Read the model definition and answer for the solid it produces. Units are mm, in the model's axes. Face numbers are marked on the shaded views. A direction names the side the tool comes from. Coordinates: 2 decimals unless noted, no trailing zeros. Order: outer loops, then holes, each group sorted by start corner. A loop starts at its lowest first (then second) coordinate and runs counter-clockwise, first axis right, second up. Notation, with made-up numbers: (-28.5, 89) -> (18.5, 89) arc R14 cw to (18.5, 104) -> close; hole circle Ø5 at (14.5, -37.75). An arc over 180 degrees is marked (long way). Answer as a JSON object with one key per item and string values. Group by question number.
1) Consider L1, parallel to Y at x = 0, z = 6; L2, parallel to X at y = 0, z = 3; L3, parallel to Z at x = -0.75, y = -2. Determine where each line is inside the solid, lowest interval first.
2) Section D-D on z = 11 is taken. Determine the outline of the cut face in (x, y), and give its area (3 significant figures).
3) A tool of negligible diameter and unlimited length cuts with its end or side. For the marked faces 4, 5 and 6, from which of +Z, -Z, +X, -X, +Y, -Y can it reach the whole face along a straight path? Write none if from no direction.
4) Given pin 1 (6 mm diameter, centred on x = 3, z = 6.5, fed in from +Y); pin 2 (7 mm diameter, centred on y = -1.5, z = 20.5, fed in from -X); pin 3 (1.5 mm diameter, centred on y = -8.5, z = 13.5, fed in from -X); pin 4 (1.5 mm diameter, centred on x = -4, y = -9.5, fed in from +Z), each flat-ended and moving along its own axis, determine where each tip first touches the part or whether it passes through.
5) Section C-C on x = 0 is taken. Determine the outline of the cut face in (y, z).
6) Section B-B on z = 19.5 is taken. Determine the outline of the cut face in (x, y).
7) Determine the mould class of the marked faces 1, 2 and 3 for opening direction X: released by +X, released by -X, zero draft, split by the parting line, or undercut.
8) Section A-A on y = 0 is taken. Determine the outline of the cut face in (x, z), and give its area (3 significant figures).
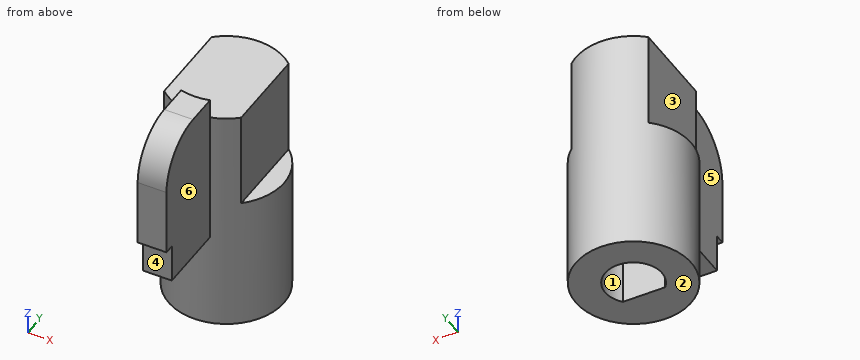
from build123d import *

# Parameters (mm, degrees)
F0_R      = 6
F1_DEPTH  = 10
F2_R      = 6
F3_DEPTH  = 6
F5_DEPTH  = 16
F7_DEPTH  = 8
F8_W      = 1
F8_H      = 4
F9_DEPTH  = 7.501
F10_DEPTH = 2


# Not quite as in the source:
# - a feature names something its author has since deleted; it is built from what else it names


with BuildPart() as f1:
    # F0 (on Top) → F1 (new body)
    with BuildSketch(Plane.XY):
        Circle(F0_R)
        with BuildLine():
            ThreePointArc((-2.1988001779, -1.9666666667), (0, 2.95), (2.1988001779, -1.9666666667))
            Line((2.1988001779, -1.9666666667), (-2.1988001779, -1.9666666667))
        make_face(mode=Mode.SUBTRACT)
    extrude(amount=F1_DEPTH)

    # F2 (on face) → F3 (join)
    with BuildSketch(Plane.XY.offset(10)):
        Circle(F2_R)
    extrude(amount=F3_DEPTH)



with BuildPart() as f5:
    # F4 (on face) → F5 (new body)
    with BuildSketch(Plane.XY.offset(10)):
        with BuildLine():
            ThreePointArc((1.5, -5.8094750193), (0, -6), (-1.5, -5.8094750193))
            Line((-1.5, -5.8094750193), (-1.5, -14))
            Line((-1.5, -14), (1.5, -14))
            Line((1.5, -14), (1.5, -5.8094750193))
        make_face()
    extrude(amount=F5_DEPTH)


with BuildPart() as f1_1:
    add(f1.part)

    add(f5.part)  # F7 merges F5
    # F6 (on face) → F7 (join)
    with BuildSketch(Plane.XY.offset(16)):
        with BuildLine():
            Line((-4, 4.472135955), (-4, -4.472135955))
            ThreePointArc((-4, -4.472135955), (0, -6), (4, -4.472135955))
            Line((4, -4.472135955), (4, 4.472135955))
            ThreePointArc((4, 4.472135955), (0, 6), (-4, 4.472135955))
        make_face()
    extrude(amount=F7_DEPTH)

    # F8 (on face) → F9 (cut, through all)
    with BuildSketch(Plane(origin=(-1.5, 0, 0), x_dir=(0, -1, 0), z_dir=(-1, 0, 0))):
        with BuildLine():
            ThreePointArc((9, 26), (12.5355339059, 24.5355339059), (14, 21))
            Line((14, 21), (14, 26))
            Line((14, 26), (9, 26))
        make_face()
        with Locations((13.5, 12)):
            Rectangle(F8_W, F8_H)
    extrude(amount=-F9_DEPTH, mode=Mode.SUBTRACT)

    # F6 (on face) → F10 (cut)
    with BuildSketch(Plane.XY.offset(16)):
        with BuildLine():
            Line((4, 4.472135955), (4, -4.472135955))
            ThreePointArc((4, -4.472135955), (5.4772255751, -2.4494897428), (6, 0))
            ThreePointArc((6, 0), (5.4772255751, 2.4494897428), (4, 4.472135955))
        make_face()
        with BuildLine():
            ThreePointArc((-4, 4.472135955), (-6, 0), (-4, -4.472135955))
            Line((-4, -4.472135955), (-4, 4.472135955))
        make_face()
    extrude(amount=-F10_DEPTH, mode=Mode.SUBTRACT)


solid = f1_1.part
Worked answers:
{
 "1": {"L1": "y = -6 to -1.97, 2.95 to 6", "L2": "x = -6 to -2.95, 2.95 to 6", "L3": "z = 0 to 24"},
 "2": {"outline": "(-1.5, -13) -> (1.5, -13) -> (1.5, -5.81) arc R6 ccw (long way) to (-1.5, -5.81) -> close", "area": "134 mm²"},
 "3": {"face 4": "-Z, +X, -X, -Y", "face 5": "+Z, -Z, -X, -Y", "face 6": "+Z, -Z, +X, -Y"},
 "4": {"pin 1": "stops at y = 6", "pin 2": "stops at x = -4", "pin 3": "stops at x = -1.5", "pin 4": "passes through"},
 "5": {"outline": "(-14, 14) -> (-13, 14) -> (-13, 10) -> (-6, 10) -> (-6, 0) -> (-1.97, 0) -> (-1.97, 10) -> (2.95, 10) -> (2.95, 0) -> (6, 0) -> (6, 24) -> (-6, 24) -> (-6, 26) -> (-9, 26) arc R5 ccw to (-14, 21) -> close"},
 "6": {"outline": "(-4, -4.47) arc R6 ccw to (-1.5, -5.81) -> (-1.5, -14) -> (1.5, -14) -> (1.5, -5.81) arc R6 ccw to (4, -4.47) -> (4, 4.47) arc R6 ccw to (-4, 4.47) -> close"},
 "7": {"face 1": "undercut", "face 2": "zero draft", "face 3": "released by -X"},
 "8": {"outline": "(-6, 0) -> (-2.95, 0) -> (-2.95, 10) -> (2.95, 10) -> (2.95, 0) -> (6, 0) -> (6, 14) -> (4, 14) -> (4, 24) -> (-4, 24) -> (-4, 14) -> (-6, 14) -> close", "area": "189 mm²"}
}
